Read the model definition and answer for the solid it produces. Units are mm, in the model's axes. Coordinates: 2 decimals unless noted, no trailing zeros. Write each loop counter-clockwise with the first axis right and the second up, starting at its lowest first coordinate (ties: lowest second). Pieces come first, ordered by that corner, then holes. Notation, with made-up numbers: (67, -8.75) -> (90, -8.75) arc R20 cw to (90, 16.25) -> close; hole circle Ø10 at (-20.75, 1). An arc over 180 degrees is marked (long way). One line per item, written item: value. Start each with the question number.
1. Find section B-B, the plane z = -53.5. Write down the section's boundary in (x, y), and give its area (3 significant figures).
2. Consider line 1 along Y through (x, z) = (1.2, 0); line 2 along Z through (x, y) = (2.55, -74.61); line 3 along Y through (x, z) = (1.05, 63). Determine where each line is inside the solid, lowest interval first.
3. Find section A-A, the plane x = 0.6. State how many separate pieces and enclosed holes the cut face has, and give its area (3 significant figures).
4. Given P1, Ø1.6, axis at x = 1.5, y = -74, coming from the -Z side; P2, Ø1.3, axis at x = 2, z = 69, coming from the -Y side; P3, Ø1.4, axis at x = 2, y = 2.5, coming from the +Z side, each flat-ended and moving along its own axis, determine where each tip first touches the part or whether it passes through.
```python
from build123d import *

# Parameters (mm, degrees)
SKETCH1_W           = 152.4
SKETCH1_H           = 146.04
BOSS_EXTRUDE1_DEPTH = 3.18
SKETCH3_R           = 1.4
SKETCH3_W           = 10
SKETCH3_H           = 3.18
BOSS_EXTRUDE5_DEPTH = 3.18
CUT_EXTRUDE2_DEPTH  = 4.18
CUT_EXTRUDE3_DEPTH  = 4.18


with BuildPart() as part:
    # Sketch1 → Boss-Extrude1 (new body)
    with BuildSketch(Plane(origin=(0, 0, 0), x_dir=(0, 0, -1), z_dir=(1, 0, 0))):
        Rectangle(SKETCH1_W, SKETCH1_H)
    extrude(amount=BOSS_EXTRUDE1_DEPTH)

    # Sketch3 → Boss-Extrude5 (add)
    with BuildSketch(Plane.ZY):
        Polygon((0, 73.02), (5, 73.02), (5, 76.2), (-5, 76.2), (-5, 73.02), align=None)
        with Locations((0, 74.61)):
            Circle(SKETCH3_R, mode=Mode.SUBTRACT)
        with Locations((0, -74.61)):
            Rectangle(SKETCH3_W, SKETCH3_H)
        with Locations((0, -74.61)):
            Circle(SKETCH3_R, mode=Mode.SUBTRACT)
    extrude(amount=-BOSS_EXTRUDE5_DEPTH)

    # Sketch4 → Cut-Extrude2 (cut, through all)
    with BuildSketch(Plane(origin=(0, 0, 0), x_dir=(0, 0, -1), z_dir=(1, 0, 0))):
        Polygon((-76.2, -5), (-76.2, 5), (-73.02, 5), (-73.02, 1.47), (-70.02, 1.47), (-70.02, 3.25), (-67.42, 3.25), (-67.42, 1.47), (-63.2, 1.47), (-63.2, -1.47), (-67.42, -1.47), (-67.42, -3.25), (-70.02, -3.25), (-70.02, -1.47), (-73.02, -1.47), (-73.02, -5), align=None)
    extrude(amount=CUT_EXTRUDE2_DEPTH, mode=Mode.SUBTRACT)

    # Sketch5 → Cut-Extrude3 (cut, through all)
    with BuildSketch(Plane.ZY):
        Polygon((-70.02, -1.47), (-73.02, -1.47), (-73.02, -5), (-76.2, -5), (-76.2, 5), (-73.02, 5), (-73.02, 1.47), (-70.02, 1.47), (-70.02, 3.25), (-67.42, 3.25), (-67.42, 1.47), (-63.2, 1.47), (-63.2, -1.47), (-67.42, -1.47), (-67.42, -3.25), (-70.02, -3.25), align=None)
    extrude(amount=-CUT_EXTRUDE3_DEPTH, mode=Mode.SUBTRACT)


solid = part.part
```
Answer block:
1. outline: (0, -73.02) -> (3.18, -73.02) -> (3.18, 73.02) -> (0, 73.02) -> close
1. area: 464 mm2
2. line 1: y = -76.2 to -76.01, -73.21 to 73.21, 76.01 to 76.2
2. line 2: z = -5 to -1.4, 1.4 to 5
2. line 3: y = -73.02 to 73.02
3. separate pieces: 1
3. enclosed holes: 2
3. area: 22,200 mm2
4. P1: stops at z = -5
4. P2: stops at y = -73.02
4. P3: stops at z = 73.02
